from build123d import *

# Parameters (mm, degrees)
SKETCH023_R     = 20
PAD008_DEPTH    = 4
SKETCH024_R     = 1.1
POCKET008_DEPTH = 5
SKETCH025_R     = 6.25
PAD009_DEPTH    = 28


with BuildPart() as part:
    # Sketch023 → Pad008 (new body)
    with BuildSketch(Plane.YZ):
        Circle(SKETCH023_R)
    extrude(amount=PAD008_DEPTH)

    # Sketch024 (on Face3 of Pad008) → Pocket008 (cut)
    with BuildSketch(Plane.YZ.offset(4)):
        with Locations((-4, 15)):
            Circle(SKETCH024_R)
        with Locations((4, 15)):
            Circle(SKETCH024_R)
        with Locations((-4, -15)):
            Circle(SKETCH024_R)
        with Locations((4, -15)):
            Circle(SKETCH024_R)
    extrude(amount=-POCKET008_DEPTH, mode=Mode.SUBTRACT)

    # Sketch025 (on Face3 of Pocket008) → Pad009 (join)
    with BuildSketch(Plane.YZ.offset(4)):
        Circle(SKETCH025_R)
    extrude(amount=PAD009_DEPTH)


with BuildPart() as part_1:
    # Body003 placement: moved
    add(part.part.moved(Location((28, 0, 65))))


solid = part_1.part
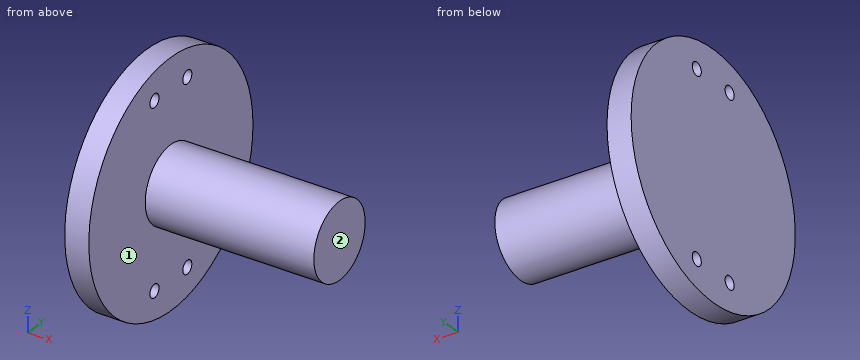
Check sheet for the modelled part. Datum: model origin and axes. Units: mm. Face numbers are marked on the shaded views. A direction names the side the tool comes from. Round coordinates to 2 decimals unless told otherwise and drop trailing zeros. Order: outer loops, then holes, each group sorted by start corner. A loop starts at its lowest first (then second) coordinate and runs counter-clockwise, first axis right, second up. Notation, with made-up numbers: M -35,-23 L 3,-23 A33 cw 3,13 Z; hole C 89.5,46.25 d5. An arc over 180 degrees is marked long. One line per item, written item: value. Start each with the question number.
1. Gauge pin test, flat ends, axial feed: P1, Ø1.5, axis at y = 3, z = 51.5, coming from the +X side; P2, Ø1.5, axis at x = 49.5, y = 1, coming from the +Z side (3 decimals); P3, Ø8, axis at x = 55, z = 61.5, coming from the -Y side. Record the tip position at first contact, or that the pin passes through.
2. Section check B-B on y = -3.5. Enter the section's corners in (x, z), and give its area (3 significant figures).
3. Scan lines: line 1 along Y through (x, z) = (30, 50); line 2 along Z through (x, y) = (29.95, -4); line 3 along X through (y, z) = (-11, 49). Record each from-to range of solid material in increasing order.
4. Section check C-C on x = 30. Enter the section's corners in (y, z).
5. Section check A-A on z = 65. Enter the section's corners in (x, y).
6. Access from +Z, -Z, +X, -X, +Y, -Y to the whole of each face (thin tool, end or side, straight path). Record for the marked faces 1 and 2.
7. Section check D-D on z = 80. Enter the section's corners in (x, y).
Results found:
1. P1: x = 32
1. P2: z = 71.245
1. P3: y = -6.25
2. outline: M 28,45.31 L 32,45.31 L 32,49.02 L 28,49.02 Z; M 28,50.98 L 32,50.98 L 32,59.82 L 60,59.82 L 60,70.18 L 32,70.18 L 32,79.02 L 28,79.02 Z; M 28,80.98 L 32,80.98 L 32,84.69 L 28,84.69 Z
2. area: 432 mm^2
3. line 1: -13.23 to -5.1, -2.9 to 2.9, 5.1 to 13.23
3. line 2: 45.4 to 48.9, 51.1 to 78.9, 81.1 to 84.6
3. line 3: 28 to 32
4. outline: C 0,65 d40; hole C -4,50 d2.2; hole C -4,80 d2.2; hole C 4,50 d2.2; hole C 4,80 d2.2
5. outline: M 28,-20 L 32,-20 L 32,-6.25 L 60,-6.25 L 60,6.25 L 32,6.25 L 32,20 L 28,20 Z
6. face 1: +X
6. face 2: +Z, -Z, +X, +Y, -Y
7. outline: M 28,-13.23 L 32,-13.23 L 32,-5.1 L 28,-5.1 Z; M 28,-2.9 L 32,-2.9 L 32,2.9 L 28,2.9 Z; M 28,5.1 L 32,5.1 L 32,13.23 L 28,13.23 Z
